CAD build for the part. Positions are in the model's coordinates, mm. Face numbers are marked on the shaded views. A direction names the side the tool comes from. Coordinates: 2 decimals unless noted, no trailing zeros. Order: outer loops, then holes, each group sorted by start corner. A loop starts at its lowest first (then second) coordinate and runs counter-clockwise, first axis right, second up. Notation, with made-up numbers: M 16.5,-13 L 30.5,-13 A20 cw 30.5,16 Z; hole C 54,-19 d5. An arc over 180 degrees is marked long. One line per item, written item: value.
from build123d import *

# Parameters (mm, degrees)
SKETCH1_W           = 60
SKETCH1_H           = 60
BOSS_EXTRUDE1_DEPTH = 15
CUT_EXTRUDE1_DEPTH  = 15
SKETCH8_W           = 15
SKETCH8_H           = 30
BOSS_EXTRUDE2_DEPTH = 100
BOSS_EXTRUDE3_DEPTH = 15
CUT_EXTRUDE4_DEPTH  = 15
FILLET1_R           = 30
FILLET3_R           = 5
FILLET4_R           = 10
FILLET5_R           = 30


with BuildPart() as part:
    # Sketch1 → Boss-Extrude1 (new body)
    with BuildSketch(Plane(origin=(0, 0, 0), x_dir=(0, 0, -1), z_dir=(1, 0, 0))):
        Rectangle(SKETCH1_W, SKETCH1_H)
    extrude(amount=BOSS_EXTRUDE1_DEPTH)

    # Sketch2 → Cut-Extrude1 (cut)
    with BuildSketch(Plane(origin=(15, 0, 0), x_dir=(0, 0, -1), z_dir=(1, 0, 0))):
        with BuildLine():
            ThreePointArc((2.5, 0), (2.236067977, 1.118033989), (1.5, 2))
            Line((1.5, 2), (-1.5, 2))
            ThreePointArc((-1.5, 2), (-1.118033989, -2.236067977), (2.5, 0))
        make_face()
    extrude(amount=-CUT_EXTRUDE1_DEPTH, mode=Mode.SUBTRACT)

    # Sketch8 → Boss-Extrude2 (add)
    with BuildSketch(Plane.XZ.offset(30)):
        with Locations((7.5, 0)):
            Rectangle(SKETCH8_W, SKETCH8_H)
    extrude(amount=BOSS_EXTRUDE2_DEPTH)

    # Sketch9 → Boss-Extrude3 (add)
    with BuildSketch(Plane.XZ.offset(130)):
        Polygon((0, 0), (0, 75), (60, 75), (60, -15), (0, -15), align=None)
    extrude(amount=BOSS_EXTRUDE3_DEPTH)

    # Sketch10 → Cut-Extrude4 (cut)
    with BuildSketch(Plane(origin=(0, -130, 0), x_dir=(1, 0, 0), z_dir=(0, 1, 0))):
        with BuildLine():
            Line((48.15, -64), (48.15, -30))
            ThreePointArc((48.15, -30), (45.5, -27.35), (42.85, -30))
            Line((42.85, -30), (42.85, -64))
            ThreePointArc((42.85, -64), (45.5, -66.65), (48.15, -64))
        make_face()
        with BuildLine():
            Line((17.15, -64), (17.15, -30))
            ThreePointArc((17.15, -30), (14.5, -27.35), (11.85, -30))
            Line((11.85, -30), (11.85, -64))
            ThreePointArc((11.85, -64), (14.5, -66.65), (17.15, -64))
        make_face()
    extrude(amount=-CUT_EXTRUDE4_DEPTH, mode=Mode.SUBTRACT)

    # Fillet1
    # the kernel refuses this fillet: 30 mm, written as the material it takes off along each edge
    with BuildSketch(Plane(origin=(-75, 30, 30), x_dir=(0, -1, 0), z_dir=(1, 0, 0))) as fillet1_piece_1:
        with BuildLine():
            CenterArc((FILLET1_R, FILLET1_R), FILLET1_R, 180, 90)
            Line((0, FILLET1_R), (-FILLET1_R * 0.02, FILLET1_R))
            Line((-FILLET1_R * 0.02, FILLET1_R), (-FILLET1_R * 0.02, -FILLET1_R * 0.02))
            Line((-FILLET1_R * 0.02, -FILLET1_R * 0.02), (FILLET1_R, -FILLET1_R * 0.02))
            Line((FILLET1_R, -FILLET1_R * 0.02), (FILLET1_R, 0))
        make_face()
    extrude(amount=165, mode=Mode.SUBTRACT)
    with BuildSketch(Plane(origin=(-64.951905284, -30, 30), x_dir=(0, 0, -1), z_dir=(1, 0, 0))) as fillet1_piece_2:
        with BuildLine():
            CenterArc((30, 25.980762114), FILLET1_R, 180, 60)
            Line((0, 25.980762114), (-0.6, 25.980762114))
            Line((-0.6, 25.980762114), (-0.6, 0))
            Line((-0.6, 0), (0, -0.6))
            ThreePointArc((0, -0.6), (7.5, -0.6), (14.7, -0.519615242))
            Line((14.7, -0.519615242), (15, 0))
        make_face()
    extrude(amount=144.903810568, mode=Mode.SUBTRACT)
    with BuildSketch(Plane(origin=(-64.951905284, -30, -30), x_dir=(0, 0, 1), z_dir=(1, 0, 0))) as fillet1_piece_3:
        with BuildLine():
            CenterArc((30, -25.980762114), FILLET1_R, 120, 60)
            Line((0, -25.980762114), (-0.6, -25.980762114))
            Line((-0.6, -25.980762114), (-0.6, 0))
            Line((-0.6, 0), (0, 0.6))
            ThreePointArc((0, 0.6), (7.5, 0.6), (14.7, 0.519615242))
            Line((14.7, 0.519615242), (15, 0))
        make_face()
    extrude(amount=144.903810568, mode=Mode.SUBTRACT)
    with BuildSketch(Plane(origin=(-75, 30, -30), x_dir=(0, -1, 0), z_dir=(1, 0, 0))) as fillet1_piece_4:
        with BuildLine():
            CenterArc((FILLET1_R, -FILLET1_R), FILLET1_R, 90, 90)
            Line((0, -FILLET1_R), (-FILLET1_R * 0.02, -FILLET1_R))
            Line((-FILLET1_R * 0.02, -FILLET1_R), (-FILLET1_R * 0.02, FILLET1_R * 0.02))
            Line((-FILLET1_R * 0.02, FILLET1_R * 0.02), (FILLET1_R, FILLET1_R * 0.02))
            Line((FILLET1_R, FILLET1_R * 0.02), (FILLET1_R, 0))
        make_face()
    extrude(amount=165, mode=Mode.SUBTRACT)

    # Fillet3
    fillet3_edges = [part.edges().sort_by_distance(p)[0] for p in [
        (15, -130, 0),
        (7.5, -130, 15),
    ]]
    fillet(fillet3_edges, radius=FILLET3_R)

    # Fillet4
    fillet4_edges = [part.edges().sort_by_distance(p)[0] for p in [
        (60, -137.5, -15),
        (60, -137.5, 75),
        (0, -137.5, 75),
    ]]
    fillet(fillet4_edges, radius=FILLET4_R)

    # Fillet5
    fillet5_edges = [part.edges().sort_by_distance(p)[0] for p in [
        (7.5, -30, -15),
        (7.5, -30, 15),
    ]]
    fillet(fillet5_edges, radius=FILLET5_R)


solid = part.part
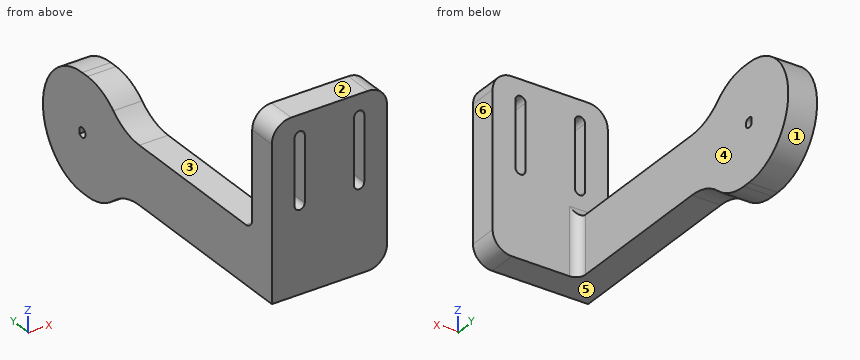
Q1. Mould opens along Y. For the marked faces 1, 2 and 3 say: released by +Y, released by -Y, zero draft, split by the parting line, or undercut.
Recorded:
face 1: released by +Y
face 2: zero draft
face 3: undercut
Q2. Drill centre lines: line 1 along X through (y, z) = (-131.5, 57.5); line 2 along Y through (x, z) = (7.5, 0); line 3 along Z through (x, y) = (23, -135). Where is each one in solid material? Low to high.
Recorded:
line 1: x = 0 to 11.85, 17.15 to 42.85, 48.15 to 60
line 2: y = -145 to -2.5, 2 to 30
line 3: z = -15 to 75
Q3. Slice it at A-A (x = 45.5). List the corners of the cut face in (y, z), plus the area to 4 significant figures.
Recorded:
outline: M -145,-15 L -130,-15 L -130,27.35 L -145,27.35 Z; M -145,66.65 L -130,66.65 L -130,75 L -145,75 Z
area: 760.5 mm^2
Q4. Slice it at C-C (x = 4.5). List the corners of the cut face in (y, z), plus the area to 3 significant figures.
Recorded:
outline: M -145,-15 L -43.71,-15 A30 cw -23.86,-22.5 A30 ccw -4.02,-30 L 0,-30 A30 ccw 0,30 L -4.02,30 A30 ccw -23.86,22.5 A30 cw -43.71,15 L -125,15 A5 cw -130,20 L -130,73.35 L -145,73.35 Z; hole M 2,-1.5 L 2,1.5 A2.5 ccw long Z
area: 7,340 mm^2
Q5. Slice it at D-D (y = -94). List the corners of the cut face in (x, z).
Recorded:
outline: M 0,-15 L 15,-15 L 15,15 L 0,15 Z
Q6. Which spindle directions (+Z, -Z, +X, -X, +Y, -Y) get a long thin tool onto all of the face, cutting with end or side? Do the marked faces 4, 5 and 6. Say none if no direction does.
Recorded:
face 4: +Z, -Z, +X, +Y
face 5: -Z, +X, -X, -Y
face 6: +Z, -Z, +X, +Y, -Y
Q7. Slice it at B-B (z = 6.5). List the corners of the cut face in (x, y).
Recorded:
outline: M 0,-145 L 60,-145 L 60,-130 L 20,-130 A5 cw 15,-125 L 15,29.29 L 0,29.29 Z
Q8. Pin check, flat tips, straight feed: pin 1 Ø6 at (y, z) = (4, 28.5) entering from -X; pin 2 Ø5 at (y, z) = (-123.5, 4) entering from +X; pin 3 Ø1 at (x, y) = (11, -68) entering from +Z; pin 4 Ø3 at (x, y) = (8.5, -1.5) entering from +Z. Stop position of each tip, or through.
Recorded:
pin 1: stops at x = 0
pin 2: stops at x = 15.1
pin 3: stops at z = 15
pin 4: stops at z = 30
